Build history of the part. All positions in model axes, mm. A direction names the side the tool comes from. Give positions to 0.01 mm unless a question says otherwise; leave off trailing zeros. Loops run counter-clockwise (first coordinate to the right, second up) from the corner with the lowest first, then second, coordinate; pieces in that order, holes last. Notation, with made-up numbers: (63.25, 41.25) - (92.25, 41.25) arc R23 ccw to (92.25, 70.25) - close; hole circle Ø7 at (52, -20.75). An arc over 180 degrees is marked (long way). Return JSON: item names as keys, results as strings. Group by question number.
1) Slice it at B-B (z = 60.5). List the corners of the cut face in (x, y), and give its area (3 significant figures).
2) Slice it at C-C (y = 5.5). Count the separate pieces of the cut face and the enclosed holes in it, and give its area (3 significant figures).
3) Slice it at A-A (x = -58). List the corners of the cut face in (y, z).
4) Drop flat-ended pins along their axis: pin 1 (8 mm diameter, centred on y = 14.5, z = 25, fed in from -X); pin 2 (12 mm diameter, centred on x = -47.5, z = 59.5, fed in from -Y); pin 3 (17.5 mm diameter, centred on x = -12, y = 12, fed in from +Z). Give the stop position or say it passes through.
5) Mould opens along Y. For faces 1 (the face through (28.378, 8.937, 74.457)), 2 (the face through (-42.41, -26.56, 16.27)), 3 (the face through (20.765, -39.923, 69.79)) say: released by +Y, released by -Y, zero draft, split by the parting line, or undercut.
6) Drill centre lines: probe 1 along Y at (x, z) = (0, 1); probe 2 along Z at (x, y) = (-9.5, -16.5); probe 3 along Z at (x, y) = (-25.5, 6.5). Where is each one in solid material? Low to high. Write a range as from..to.
7) 3-axis set-ups, long thin cutter, end or side, ignore diameter. For faces 4 (the face through (-8.67, -39.05, 1.48)), 5 (the face through (-0.3, -42.5, 16.3)), 6 (the face through (-20.633, -15.821, 42.294)), 7 (the face through (0.3, 42.5, 16.3)), 8 (the face through (42.41, 26.56, 16.27)): which of +Z, -Z, +X, -X, +Y, -Y reach the whole face in a straight line?
```python
from build123d import *

# Parameters (mm, degrees)
F1_DEPTH  = 33
F3_R      = 40
F4_DEPTH  = 3
F6_R      = 45
F6_R_2    = 34.1243185103
F7_DEPTH  = 38
F8_R      = 45
F8_R_2    = 39
F9_DEPTH  = 8
F10_R     = 31
F11_DEPTH = 30
F11_TAPER = 3.85
F12_R     = 26
F13_DEPTH = 42


with BuildPart() as f1:
    # F0 (on Top) → F1 (new body)
    with BuildSketch(Plane.XY):
        with BuildLine():
            ThreePointArc((-42.0797413793, -5.9619934125), (-42.5, 0), (-42.0797413793, 5.9619934125))
            ThreePointArc((-42.0797413793, 5.9619934125), (-51.7160080676, 15.7959312924), (-65.474137931, 15.2688330329))
            Line((-65.474137931, 15.2688330329), (-65.474137931, 0.6223039353))
            ThreePointArc((-65.474137931, 0.6223039353), (-57.6885794505, 7.4935316935), (-50.5, 0))
            ThreePointArc((-50.5, 0), (-57.6885794505, -7.4935316935), (-65.474137931, -0.6223039353))
            Line((-65.474137931, -0.6223039353), (-65.474137931, -15.2688330329))
            ThreePointArc((-65.474137931, -15.2688330329), (-51.7160080676, -15.7959312924), (-42.0797413793, -5.9619934125))
        make_face()
        with BuildLine():
            ThreePointArc((-18.6853448276, -38.1720825824), (-34.3870816807, -24.9755603237), (-42.0797413793, -5.9619934125))
            ThreePointArc((-42.0797413793, -5.9619934125), (-51.7160080676, -15.7959312924), (-65.474137931, -15.2688330329))
            Line((-65.474137931, -15.2688330329), (-18.6853448276, -38.1720825824))
        make_face()
        with BuildLine():
            Line((-65.474137931, 0.6223039353), (-65.474137931, 15.2688330329))
            ThreePointArc((-65.474137931, 15.2688330329), (-75, 0), (-65.474137931, -15.2688330329))
            Line((-65.474137931, -15.2688330329), (-65.474137931, -0.6223039353))
            ThreePointArc((-65.474137931, -0.6223039353), (-65.5, 0), (-65.474137931, 0.6223039353))
        make_face()
        with BuildLine():
            Line((65.474137931, 15.2688330329), (18.6853448276, 38.1720825824))
            ThreePointArc((18.6853448276, 38.1720825824), (34.3870816807, 24.9755603237), (42.0797413793, 5.9619934125))
            ThreePointArc((42.0797413793, 5.9619934125), (51.7160080676, 15.7959312924), (65.474137931, 15.2688330329))
        make_face()
        with BuildLine():
            ThreePointArc((75, 0), (72.4232511042, 8.9983235987), (65.474137931, 15.2688330329))
            Line((65.474137931, 15.2688330329), (65.474137931, 0.6223039353))
            ThreePointArc((65.474137931, 0.6223039353), (65.4935316935, 0.3114205495), (65.5, 0))
            ThreePointArc((65.5, 0), (65.4935316935, -0.3114205495), (65.474137931, -0.6223039353))
            Line((65.474137931, -0.6223039353), (65.474137931, -15.2688330329))
            ThreePointArc((65.474137931, -15.2688330329), (72.4232511042, -8.9983235987), (75, 0))
        make_face()
        with BuildLine():
            ThreePointArc((42.0797413793, 5.9619934125), (34.3870816807, 24.9755603237), (18.6853448276, 38.1720825824))
            ThreePointArc((18.6853448276, 38.1720825824), (0, 42.5), (-18.6853448276, 38.1720825824))
            ThreePointArc((-18.6853448276, 38.1720825824), (-34.3870816807, 24.9755603237), (-42.0797413793, 5.9619934125))
            ThreePointArc((-42.0797413793, 5.9619934125), (-41.2721131557, 3.0294886902), (-41, 0))
            ThreePointArc((-41, 0), (-41.2721131557, -3.0294886902), (-42.0797413793, -5.9619934125))
            ThreePointArc((-42.0797413793, -5.9619934125), (-34.3870816807, -24.9755603237), (-18.6853448276, -38.1720825824))
            ThreePointArc((-18.6853448276, -38.1720825824), (0, -42.5), (18.6853448276, -38.1720825824))
            ThreePointArc((18.6853448276, -38.1720825824), (34.3870816807, -24.9755603237), (42.0797413793, -5.9619934125))
            ThreePointArc((42.0797413793, -5.9619934125), (41, 0), (42.0797413793, 5.9619934125))
        make_face()
        with BuildLine():
            ThreePointArc((42.5, 0), (42.3948051571, 2.9883934965), (42.0797413793, 5.9619934125))
            ThreePointArc((42.0797413793, 5.9619934125), (41, 0), (42.0797413793, -5.9619934125))
            ThreePointArc((42.0797413793, -5.9619934125), (42.3948051571, -2.9883934965), (42.5, 0))
        make_face()
        with BuildLine():
            ThreePointArc((65.474137931, 15.2688330329), (51.7160080676, 15.7959312924), (42.0797413793, 5.9619934125))
            ThreePointArc((42.0797413793, 5.9619934125), (42.3948051571, 2.9883934965), (42.5, 0))
            ThreePointArc((42.5, 0), (42.3948051571, -2.9883934965), (42.0797413793, -5.9619934125))
            ThreePointArc((42.0797413793, -5.9619934125), (51.7160080676, -15.7959312924), (65.474137931, -15.2688330329))
            Line((65.474137931, -15.2688330329), (65.474137931, -0.6223039353))
            ThreePointArc((65.474137931, -0.6223039353), (50.5, 0), (65.474137931, 0.6223039353))
            Line((65.474137931, 0.6223039353), (65.474137931, 15.2688330329))
        make_face()
        with BuildLine():
            ThreePointArc((65.474137931, -15.2688330329), (51.7160080676, -15.7959312924), (42.0797413793, -5.9619934125))
            ThreePointArc((42.0797413793, -5.9619934125), (34.3870816807, -24.9755603237), (18.6853448276, -38.1720825824))
            Line((18.6853448276, -38.1720825824), (65.474137931, -15.2688330329))
        make_face()
        with BuildLine():
            ThreePointArc((-42.0797413793, 5.9619934125), (-34.3870816807, 24.9755603237), (-18.6853448276, 38.1720825824))
            Line((-18.6853448276, 38.1720825824), (-65.474137931, 15.2688330329))
            ThreePointArc((-65.474137931, 15.2688330329), (-51.7160080676, 15.7959312924), (-42.0797413793, 5.9619934125))
        make_face()
        with BuildLine():
            ThreePointArc((-41, 0), (-41.2721131557, 3.0294886902), (-42.0797413793, 5.9619934125))
            ThreePointArc((-42.0797413793, 5.9619934125), (-42.5, 0), (-42.0797413793, -5.9619934125))
            ThreePointArc((-42.0797413793, -5.9619934125), (-41.2721131557, -3.0294886902), (-41, 0))
        make_face()
    extrude(amount=F1_DEPTH)

    # F3 (on face) → F4 (cut)
    with BuildSketch(Plane.XY):
        Circle(F3_R)
    extrude(amount=F4_DEPTH, mode=Mode.SUBTRACT)

    # F2 (on Front) → F5 (revolve)
    with BuildSketch(Plane.XZ):
        with BuildLine():
            Line((-42.499996424, 32.9825655057), (0, 33))
            Line((0, 33), (0, 55))
            Line((0, 55), (-27.083222819, 55))
            Line((-27.083222819, 55), (-34.1243185103, 55))
            ThreePointArc((-34.1243185103, 55), (-31.4867427552, 51.7572794356), (-32.2335459741, 47.6445762521))
            Line((-32.2335459741, 47.6445762521), (-42.499996424, 32.9825655057))
        make_face()
    revolve(axis=Axis((0, 0, 44), (0, 0, 1)))

    # F6 (on face) → F7 (join)
    with BuildSketch(Plane.XY.offset(55)):
        Circle(F6_R)
        Circle(F6_R_2, mode=Mode.SUBTRACT)
        Circle(F6_R_2)
    extrude(amount=F7_DEPTH)

    # F8 (on face) → F9 (cut)
    with BuildSketch(Plane.XY.offset(93)):
        Circle(F8_R)
        Circle(F8_R_2, mode=Mode.SUBTRACT)
    extrude(amount=-F9_DEPTH, mode=Mode.SUBTRACT)

    # F10 (on face) → F11 (cut)
    with BuildSketch(Plane.XY.offset(93)):
        Circle(F10_R)
    extrude(amount=-F11_DEPTH, taper=F11_TAPER, mode=Mode.SUBTRACT)

    # F12 (on face) → F13 (cut)
    with BuildSketch(Plane.XY.offset(63)):
        Circle(F12_R)
    extrude(amount=-F13_DEPTH, mode=Mode.SUBTRACT)


solid = f1.part
```
Results:
{
 "1": {"outline": "circle Ø90 at (0, 0); hole circle Ø52 at (0, 0)", "area": "4,240 mm2"},
 "2": {"separate pieces": "3", "enclosed holes": "0", "area": "4,920 mm2"},
 "3": {"outline": "(-18.93, 0) - (-7.5, 0) - (-7.5, 33) - (-18.93, 33) - close; (7.5, 0) - (18.93, 0) - (18.93, 33) - (7.5, 33) - close"},
 "4": {"pin 1": "x = -71.37", "pin 2": "y = -17.4", "pin 3": "z = 21"},
 "5": {"face 1": "undercut", "face 2": "released by -Y", "face 3": "split by the parting line"},
 "6": {"probe 1": "-42.5..-40, 40..42.5", "probe 2": "3..21", "probe 3": "3..63"},
 "7": {"face 4": "-Z", "face 5": "-Z, -Y", "face 6": "+Z", "face 7": "-Z, +Y", "face 8": "-Z, +X, +Y"}
}
